The drawing under review shows one solid part. Ordinate dimensions are in mm from its lowest x, y, z. A direction names the side the tool comes from. Coordinates: 2 decimals unless noted, no trailing zeros. Write each loop counter-clockwise with the first axis right and the second up, starting at its lowest first coordinate (ties: lowest second). Pieces come first, ordered by that corner, then holes. Notation, with made-up numbers: (49, 6) -> (104, 6) arc R25 ccw to (104, 27) -> close; hole circle Ø4 at (30, 24.25). An arc over 180 degrees is marked (long way). One line per item, written item: value. Start each with the question number.
1) For probe 1 along Y at (x, z) = (15.05, 2.45); probe 2 along Z at (x, y) = (21, 8); probe 3 along Y at (x, z) = (14, 12.25), list the stretches that pass through material, from the lowest coordinate up. Write a range as from..to.
2) Add section B-B (x = 15.05). State the section outline as (y, z) points, and give its area (3 significant figures).
3) For pin 1 Ø5 at (y, z) = (9.5, 7) entering from +X; pin 2 Ø3 at (x, y) = (4, 20) entering from +Z; pin 3 Ø4 at (x, z) = (13, 8.5) entering from -Y; pin 4 Ø3 at (x, z) = (6.5, 5) entering from -Y, all flat-tipped, find the tip position at first contact; note any pin that passes through.
4) Mouldability with a two-part tool opening along X and no side actions: class the marked faces 3, 4, 5 and 6 as released by +X, released by -X, zero draft, split by the parting line, or undercut.
5) Add section A-A (y = 19.6). State the section outline as (x, z) points, and give its area (3 significant figures).
6) Add section D-D (x = 4.5). State the section outline as (y, z) points.
7) Machinability: for the marked faces 1 and 2, which of the approach directions +Z, -Z, +X, -X, +Y, -Y give a long, thin tool a straight path to every point of the face, cutting with its end or side? Answer none if there is none.
8) Add section C-C (z = 2.5). State the section outline as (x, y) points, and give its area (3 significant figures).
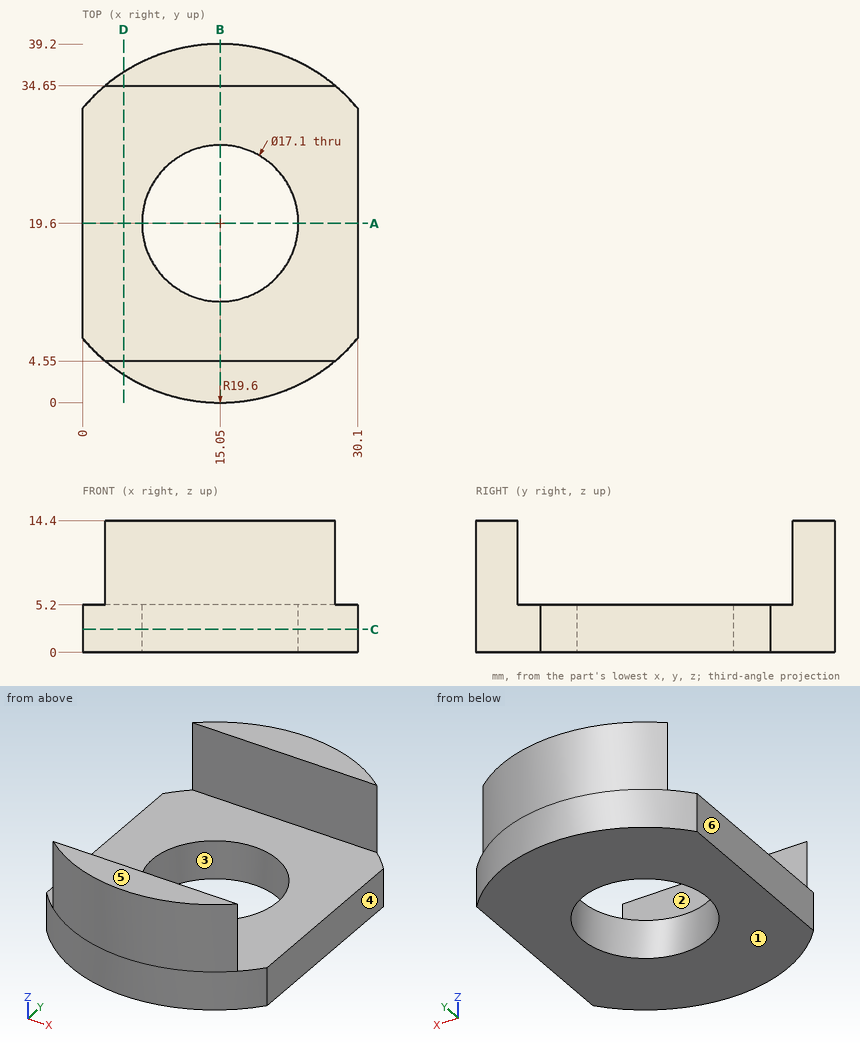
Numbers:
1. probe 1: 0..11.05, 28.15..39.2
1. probe 2: 0..5.2
1. probe 3: 0.03..4.55, 34.65..39.17
2. outline: (0, 0) -> (11.05, 0) -> (11.05, 5.2) -> (4.55, 5.2) -> (4.55, 14.4) -> (0, 14.4) -> close; (28.15, 0) -> (39.2, 0) -> (39.2, 14.4) -> (34.65, 14.4) -> (34.65, 5.2) -> (28.15, 5.2) -> close
2. area: 199 mm²
3. pin 1: x = 30.1
3. pin 2: z = 5.2
3. pin 3: y = 0
3. pin 4: y = 1.31
4. face 3: undercut
4. face 4: released by +X
4. face 5: zero draft
4. face 6: released by -X
5. outline: (0, 0) -> (6.5, 0) -> (6.5, 5.2) -> (0, 5.2) -> close; (23.6, 0) -> (30.1, 0) -> (30.1, 5.2) -> (23.6, 5.2) -> close
5. area: 67.6 mm²
6. outline: (3.08, 0) -> (36.12, 0) -> (36.12, 14.4) -> (34.65, 14.4) -> (34.65, 5.2) -> (4.55, 5.2) -> (4.55, 14.4) -> (3.08, 14.4) -> close
7. face 1: -Z, +X, -X, +Y, -Y
7. face 2: +Z, +X, -X
8. outline: (0, 7.04) arc R19.6 ccw to (30.1, 7.04) -> (30.1, 32.16) arc R19.6 ccw to (0, 32.16) -> close; hole circle Ø17.1 at (15.05, 19.6)
8. area: 821 mm²
